The figure shows three views and two pictorial views of one solid part (mm, origin at its lowest corner). Answer the questions. Give positions to 0.01 mm unless a question says otherwise; leave off trailing zeros. Write each loop counter-clockwise with the first axis right and the second up, starting at its lowest first coordinate (ties: lowest second). Pieces come first, ordered by that corner, then holes. Notation, with made-up numbers: M 3.5,66.25 L 43.5,66.25 A28 ccw 43.5,85.25 Z; hole C 62.5,-8 d2. An arc over 180 degrees is marked long. Return JSON: item names as keys, results as strings.
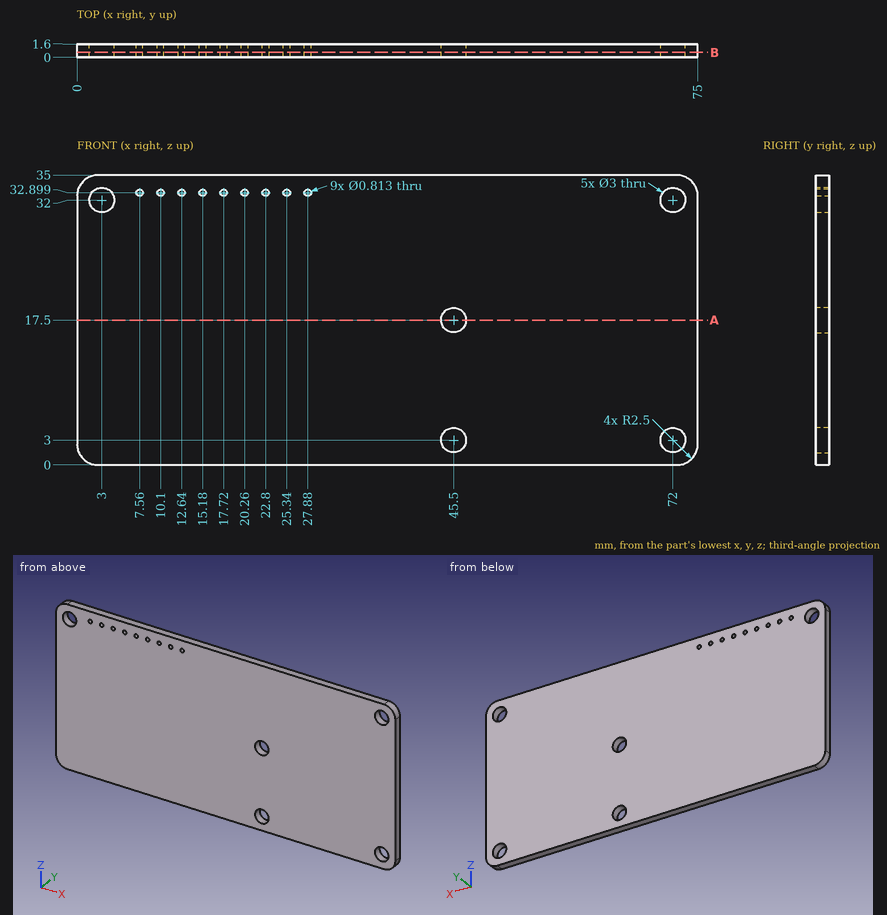
Item 1: A cutting plane is placed at B-B, the plane y = 0.6. Count the separate pieces of the cut face and the enclosed holes in it, plus the area to 3 significant figures.
Geometry results:
{"separate pieces": "1", "enclosed holes": "14", "area": "2,580 mm2"}
Item 2: A cutting plane is placed at A-A, the plane z = 17.5. Write down the section's boundary in (x, y), plus the area to 3 significant figures.
Geometry results:
{"outline": "M 0,0 L 44,0 L 44,1.6 L 0,1.6 Z; M 47,0 L 75,0 L 75,1.6 L 47,1.6 Z", "area": "115 mm2"}
Item 3: Find the intervals of material crossed by line 1 (Z direction, x = 72, y = 0.5); line 2 (X direction, y = 0.6, z = 16.5), in increasing order.
Geometry results:
{"line 1": "z = 0 to 1.5, 4.5 to 30.5, 33.5 to 35", "line 2": "x = 0 to 44.38, 46.62 to 75"}
